Source: CAD feature listing. Evaluate the final solid. Frame: model axes, mm. Face numbers are marked on the shaded views. A direction names the side the tool comes from. Give positions to 0.01 mm unless a question says otherwise; leave off trailing zeros. Write each loop counter-clockwise with the first axis right and the second up, starting at its lowest first coordinate (ties: lowest second). Pieces come first, ordered by that corner, then holes.
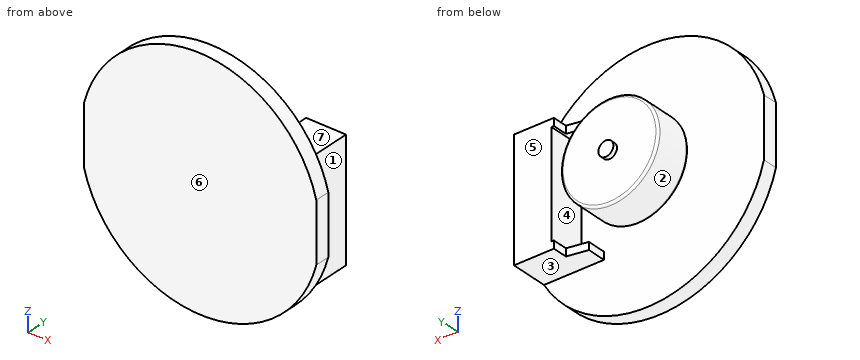
Autodesk Inventor part; units mm, degrees
ref_plane "YZ Plane" through (0, 0, 0) normal (1, 0, 0) x (0, 1, 0)
ref_plane "XZ Plane" through (0, 0, 0) normal (0, 1, 0) x (-1, 0, 0)
ref_plane "XY Plane" through (0, 0, 0) normal (0, 0, 1) x (1, 0, 0)
sketch "Эскиз1" plane through (0, 0, 0) normal (0, 1, 0) x (-1, 0, 0)
  circle A0 centre (0, 0) radius 16
  line L0 (15.5, 3.9686) -> (15.5, -3.9686)
  line L1 (-15.5, 3.9686) -> (-15.5, -3.9686)
  dimension "d0" = 32
  dimension "d1" = 15.5
  dimension "d2" = 15.5
extrude "Выдавливание1" add sketch "Эскиз1" along normal blind 2 contours L0 A0 L1
sketch "Эскиз2" plane through (0, 2, 0) normal (0, 1, 0) x (1, 0, 0)
  circle A0 centre (0, 0) radius 1
  dimension "d5" = 2
extrude "Выдавливание2" add sketch "Эскиз2" along normal blind 7
ref_plane "РабПлоскость1" through (0, 8.4, 0) normal (0, 1, 0) x (1, 0, 0)
sketch "Эскиз3" plane through (0, 8.4, 0) normal (0, 1, 0) x (1, 0, 0)
  circle A0 centre (0, 0) radius 1
  circle A1 centre (0, 0) radius 6.5
  dimension "d9" = 13
extrude "Выдавливание3" add sketch "Эскиз3" against normal blind 5
fillet "Сопряжение1" radius 0.3 2 edges at (-6.5, 8.4, 0) (-6.5, 3.4, 0)
sketch "Эскиз4" plane through (0, 2, 0) normal (0, 1, 0) x (1, 0, 0)
  line L0 (13.8564, -8) -> (5.8564, -8)
  line L1 (5.8564, -8) -> (5.8564, 8)
  line L2 (5.8564, 8) -> (13.8564, 8)
  line L3 (13.8564, 8) -> (13.8564, -8)
  arc A0 (-15.5, -3.9686) -> (15.5, -3.9686) centre (0, 0) ccw
  arc A1 (15.5, 3.9686) -> (-15.5, 3.9686) centre (0, 0) ccw
  line L4 (5.8564, -7) -> (8.8564, -7)
  line L5 (8.8564, -7) -> (8.8564, 7)
  line L6 (8.8564, 7) -> (5.8564, 7)
  line L7 (5.8564, 7) -> (5.8564, -7)
  line L8 (13.8564, 0) -> (12.4148, 0) construction
  dimension "d13" = 8
  dimension "d14" = 16
  dimension "d21" = 5
  dimension "d22" = 14
extrude "Выдавливание4" add sketch "Эскиз4" along normal blind 5 contours L0 L1 L4 L5 L6 L2 L3
sketch "Эскиз6" plane through (5.8564, 2, 8) normal (0, 0, 1) x (1, 0, 0)
  line L0 (0, 0) -> (0, 5)
  line L1 (0, 0) -> (0, 2.5)
  line L2 (0, 2.5) -> (2.6743, 3)
  line L3 (2.6743, 3) -> (2.6743, 5)
  line L4 (8, 5) -> (0, 5)
  point P0 (-5.8564, -2)
  dimension "d23" = 2.5
  dimension "d24" = 2
extrude "Выдавливание6" cut sketch "Эскиз6" against normal blind 5
mirror "Зеркальное отражение1" about plane through (0, 0, 0) normal (0, 0, 1) of "Выдавливание6"
properties part number "encoder"
1. Section query B-B (y = 3). Return loops of the section in (x, z), plus the area to 3 significant figures.
2. Line query: probe 1 along Y at (x, z) = (0, -4); probe 2 along X at (y, z) = (2.25, 0); probe 3 along Y at (x, z) = (-9.5, 9). Output: solid intervals per line, ascending.
3. Pin query (flat end, axial travel): P1, Ø1.5, axis at x = 9, y = 4, coming from the +Z side; P2, Ø0.9, axis at x = 8, y = 3.5, coming from the -Z side; P3, Ø3, axis at x = 0.5, y = 2, coming from the +Z side; P4, Ø0.5, axis at y = 5.5, z = 7.5, coming from the -X side. Return the tip coordinate at first contact, or that it passes through.
4. Section query C-C (z = 0). Return loops of the section in (x, y).
5. Access query for the marked faces 4, 5, 6 and 7. Directions: +Z, -Z, +X, -X, +Y, -Y. A direction counts if a zero-diameter tool reaches every point of the face in a straight line with its end or side. Return the directions, or none.
6. Section query D-D (x = 0). Return loops of the section in (y, z).
7. Pull-direction query (X, two-part tool) for the marked faces 1, 2 and 3; classes: pulls with the +X half, pulls with the -X half, needs draft (parallel to the pull), parting line crosses it, or undercut.
8. Section query A-A (y = 6.25). Return loops of the section in (x, z), plus the area to 3 significant figures.
The answers:
1. outline: circle Ø2 at (0, 0); (5.86, -8) - (13.86, -8) - (13.86, 8) - (5.86, 8) - (5.86, 7) - (8.86, 7) - (8.86, -7) - (5.86, -7) - close
1. area: 89.1 mm2
2. probe 1: y = 0 to 2, 3.4 to 8.4
2. probe 2: x = -1 to 1, 8.86 to 13.86
2. probe 3: y = 0 to 2
3. P1: stops at z = 8
3. P2: stops at z = -8
3. P3: stops at z = 16
3. P4: stops at x = 8.53
4. outline: (-15.5, 0) - (15.5, 0) - (15.5, 2) - (13.86, 2) - (13.86, 7) - (8.86, 7) - (8.86, 2) - (1, 2) - (1, 3.4) - (6.2, 3.4) arc R0.3 ccw to (6.5, 3.7) - (6.5, 8.1) arc R0.3 ccw to (6.2, 8.4) - (1, 8.4) - (1, 9) - (-1, 9) - (-1, 8.4) - (-6.2, 8.4) arc R0.3 ccw to (-6.5, 8.1) - (-6.5, 3.7) arc R0.3 ccw to (-6.2, 3.4) - (-1, 3.4) - (-1, 2) - (-15.5, 2) - close
5. face 4: +Y
5. face 5: +Z, -Z, +X, +Y
5. face 6: +Z, -Z, +X, -X, -Y
5. face 7: +Z, +X, -X, +Y
6. outline: (0, -16) - (2, -16) - (2, -1) - (3.4, -1) - (3.4, -6.2) arc R0.3 ccw to (3.7, -6.5) - (8.1, -6.5) arc R0.3 ccw to (8.4, -6.2) - (8.4, -1) - (9, -1) - (9, 1) - (8.4, 1) - (8.4, 6.2) arc R0.3 ccw to (8.1, 6.5) - (3.7, 6.5) arc R0.3 ccw to (3.4, 6.2) - (3.4, 1) - (2, 1) - (2, 16) - (0, 16) - close
7. face 1: pulls with the +X half
7. face 2: undercut
7. face 3: needs draft
8. outline: circle Ø13 at (0, 0); (8.53, -8) - (13.86, -8) - (13.86, 8) - (8.53, 8) - (8.53, 7) - (8.86, 7) - (8.86, -7) - (8.53, -7) - close
8. area: 213 mm2
